Print and shaded views of the part. All mm, measured from the part's lowest x, y and z. Round coordinates to 2 decimals unless told otherwise and drop trailing zeros. Loops run counter-clockwise (first coordinate to the right, second up) from the corner with the lowest first, then second, coordinate; pieces in that order, holes last. Notation, with made-up numbers: (89.5, 86.25) - (129.5, 86.25) arc R14 cw to (129.5, 111.25) - close; hole circle Ø6 at (87, 29). An arc over 180 degrees is marked (long way). Use one line per item in the form item = value.
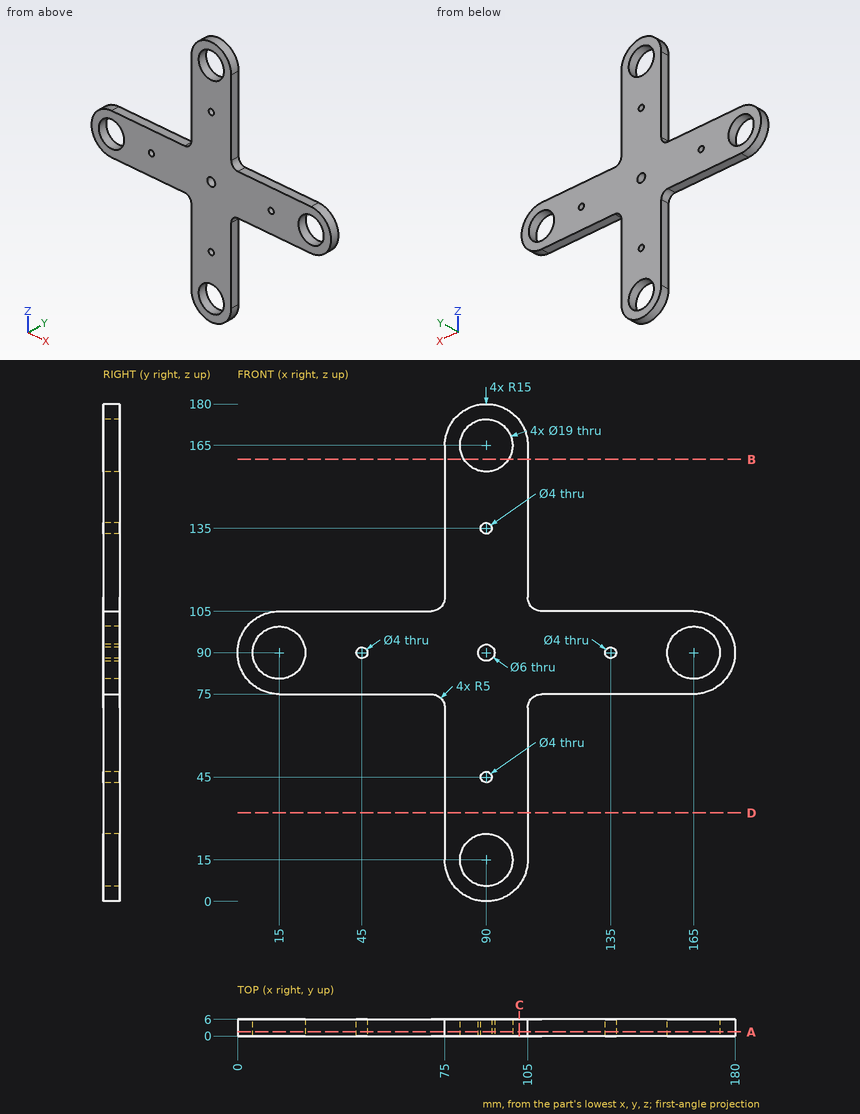
1) Slice it at A-A (y = 1.45). State how many separate pieces and enclosed holes the cut face has, plus the area to 3 significant figures.
Report:
separate_pieces = 1
enclosed_holes = 9
area = 8,320 mm^2
2) Drill centre lines: probe 1 along Z at (x, y) = (90, 2); probe 2 along Z at (x, y) = (96.5, 3.8); probe 3 along X at (y, z) = (3.65, 135). Where is each one in solid material? Low to high.
Report:
probe_1 = 0 to 5.5, 24.5 to 43, 47 to 87, 93 to 133, 137 to 155.5, 174.5 to 180
probe_2 = 1.48 to 8.07, 21.93 to 158.07, 171.93 to 178.52
probe_3 = 75 to 88, 92 to 105
3) Slice it at B-B (z = 160). Write the cut outline in (x, y), plus the area to 3 significant figures.
Report:
outline = (75, 0) - (81.92, 0) - (81.92, 6) - (75, 6) - close; (98.08, 0) - (105, 0) - (105, 6) - (98.08, 6) - close
area = 83.1 mm^2
4) Flat gauge pins, fed straight in: pin 1 (1.8 mm diameter, centred on y = 2, z = 146.5, fed in from -X); pin 2 (3 mm diameter, centred on x = 102.5, y = 2.5, fed in from +Z); pin 3 (2.5 mm diameter, centred on x = 135, z = 90, fed in from +Y); pin 4 (1 mm diameter, centred on x = 67, y = 1.5, fed in from -Z). Where does each tip first touch, or does it go through?
Report:
pin_1 = 75
pin_2 = 175.2
pin_3 = through
pin_4 = 75
5) Slice it at D-D (z = 32). Write the cut outline in (x, y).
Report:
outline = (75, 0) - (105, 0) - (105, 6) - (75, 6) - close
6) Slice it at C-C (x = 102). Write the cut outline in (y, z).
Report:
outline = (0, 6) - (6, 6) - (6, 174) - (0, 174) - close
